Autodesk Inventor part; units mm, degrees
ref_plane "YZ Plane" through (0, 0, 0) normal (1, 0, 0) x (0, 1, 0)
ref_plane "XZ Plane" through (0, 0, 0) normal (0, 1, 0) x (-1, 0, 0)
ref_plane "XY Plane" through (0, 0, 0) normal (0, 0, 1) x (1, 0, 0)
sketch "Sketch1" plane through (0, 0, 0) normal (0, 1, 0) x (-1, 0, 0)
  line L0 (0, 0) -> (0, -20)
  line L1 (0, -20) -> (3, -20)
  line L2 (3, -20) -> (3, -30)
  line L3 (3, -30) -> (0, -30)
  line L4 (0, -30) -> (0, -50)
  line L5 (0, -50) -> (-17, -50)
  line L6 (-17, -50) -> (-17, -47)
  line L7 (-17, -47) -> (-27, -47)
  line L8 (-27, -47) -> (-27, -50)
  line L9 (-27, -50) -> (-44, -50)
  line L10 (-44, -50) -> (-44, -30)
  line L11 (-44, -30) -> (-47, -30)
  line L12 (-47, -30) -> (-47, -20)
  line L13 (-47, -20) -> (-44, -20)
  line L14 (-44, -20) -> (-44, 0)
  line L15 (0, 0) -> (-17, 0)
  line L16 (-17, 0) -> (-17, -3)
  line L17 (-17, -3) -> (-27, -3)
  line L18 (-27, -3) -> (-27, 0)
  line L19 (-27, 0) -> (-44, 0)
  circle A0 centre (-22, -25) radius 2.5
  point P0 (3, -25)
  point P1 (-22, -3)
  dimension "d5" = 3
  dimension "d7" = 10
  dimension "d8" = 3
  dimension "d9" = 50
  dimension "d10" = 10
  dimension "d11" = 50
  dimension "d14" = 5
extrude "Extrusion2" add sketch "Sketch1" along normal blind 3
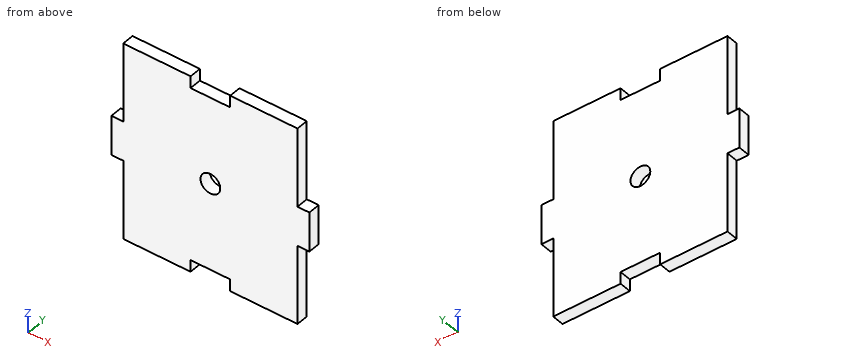
Model file for the job. Use its own axes, mm. Round coordinates to 2 decimals unless told otherwise and drop trailing zeros. Order: outer loops, then holes, each group sorted by start corner. A loop starts at its lowest first (then second) coordinate and runs counter-clockwise, first axis right, second up.
(1) Drill centre lines: line 1 (Z direction, x = 22, y = 2); line 2 (X direction, y = 0.75, z = -13); line 3 (Z direction, x = 25.5, y = 2.65). Where is each one in solid material? Low to high.
(2) Band-saw the part on A-A (z = -25). List the corners of the cut face in (x, y), then the cut area to 3 significant figures.
(3) Band-saw the part on B-B (x = 22). List the corners of the cut face in (y, z), then the cut area to 3 significant figures.
(4) Pin check, flat tips, straight feed: pin 1 (1.5 mm diameter, centred on y = 2, z = -38, fed in from +X); pin 2 (1.5 mm diameter, centred on x = -1.5, y = 1, fed in from -Z); pin 3 (1.5 mm diameter, centred on y = 1.5, z = -43, fed in from -X). Stop position of each tip, or through.
(5) Band-saw the part on D-D (z = -36). List the corners of the cut face in (x, y), then the cut area to 3 significant figures.
(6) Band-saw the part on C-C (y = 1.1). List the corners of the cut face in (x, z).
Verdict:
1. line 1: z = -47 to -27.5, -22.5 to -3
1. line 2: x = 0 to 44
1. line 3: z = -47 to -3
2. outline: (-3, 0) - (19.5, 0) - (19.5, 3) - (-3, 3) - close; (24.5, 0) - (47, 0) - (47, 3) - (24.5, 3) - close
2. area: 135 mm2
3. outline: (0, -47) - (3, -47) - (3, -27.5) - (0, -27.5) - close; (0, -22.5) - (3, -22.5) - (3, -3) - (0, -3) - close
3. area: 117 mm2
4. pin 1: stops at x = 44
4. pin 2: stops at z = -30
4. pin 3: stops at x = 0
5. outline: (0, 0) - (44, 0) - (44, 3) - (0, 3) - close
5. area: 132 mm2
6. outline: (-3, -30) - (0, -30) - (0, -50) - (17, -50) - (17, -47) - (27, -47) - (27, -50) - (44, -50) - (44, -30) - (47, -30) - (47, -20) - (44, -20) - (44, 0) - (27, 0) - (27, -3) - (17, -3) - (17, 0) - (0, 0) - (0, -20) - (-3, -20) - close; hole circle Ø5 at (22, -25)
